The model under review builds one solid part; all positions refer to its coordinate system, in mm. Give positions to 0.01 mm unless a question says otherwise; leave off trailing zeros. Write each loop counter-clockwise with the first axis right and the second up, starting at its lowest first coordinate (ties: lowest second). Pieces come first, ordered by that corner, then holes. Notation, with made-up numbers: (-14, -35) - (-4, -35) arc R14 cw to (-4, -18) - close; hole circle Ø2 at (42, -35). An arc over 180 degrees is marked (long way). Write item = value, one per line.
```python
from build123d import *

# Parameters (mm, degrees)
EXTRUDE_THIN1_DEPTH = 1.2
EXTRUDE_THIN2_DEPTH = 1.2
BOSS_EXTRUDE1_DEPTH = 50.02
EXTRUDE_THIN5_START = -2.6
EXTRUDE_THIN5_DEPTH = 2.6


# Read off the part's stored shape, not the designer's step: Extrude-Thin1
with BuildPart() as part:
    # Extrude-Thin1 outline → Extrude-Thin1 (new body)
    with BuildSketch(Plane(origin=(0, 0, 0), x_dir=(1, 0, 0), z_dir=(0, 1, 0))):
        Polygon((-25.01, 39.998768944), (-15.007807764, -0.01), (15.007807764, -0.01), (25.01, 39.998768944), (25.01, 42.01), (-25.01, 42.01), align=None)
        Polygon((13.594602468, 1.8), (-13.594602468, 1.8), (-23.194602468, 40.2), (23.194602468, 40.2), align=None, mode=Mode.SUBTRACT)
    extrude(amount=EXTRUDE_THIN1_DEPTH)

    # Sketch3 → Extrude-Thin2 (add)
    with BuildSketch(Plane.XZ):
        Polygon((23.844483111, -39.577380413), (-12.944721826, -1.177380413), (-14.244483111, -2.422619587), (22.544721826, -40.822619587), align=None)
        Polygon((-22.544721826, -40.822619587), (14.244483111, -2.422619587), (12.944721826, -1.177380413), (-23.844483111, -39.577380413), align=None)
    extrude(amount=-EXTRUDE_THIN2_DEPTH)

    # Sketch4 → Boss-Extrude1 (add)
    with BuildSketch(Plane.ZY.offset(25.01)):
        with BuildLine():
            Line((-42.326963696, 2.62973084), (-42.83410561, 3.717300185))
            ThreePointArc((-42.83410561, 3.717300185), (-43.913777214, 1.527942753), (-42.01, 0))
            Line((-42.01, 0), (-42.01, 1.2))
            ThreePointArc((-42.01, 1.2), (-42.742222005, 1.78767029), (-42.326963696, 2.62973084))
        make_face()
    extrude(amount=-BOSS_EXTRUDE1_DEPTH)

    # Sketch5 → Extrude-Thin5 (add)
    with BuildSketch(Plane.XZ.offset(EXTRUDE_THIN5_START)):
        Polygon((25.01, -42.01), (25.01, -39.998768944), (15.007807764, 0.01), (-15.007807764, 0.01), (-25.01, -39.998768944), (-25.01, -42.01), (-25.81, -42.01), (-25.81, -39.900284443), (-15.632428889, 0.81), (15.632428889, 0.81), (25.81, -39.900284443), (25.81, -42.01), align=None)
    extrude(amount=EXTRUDE_THIN5_DEPTH)


solid = part.part
```
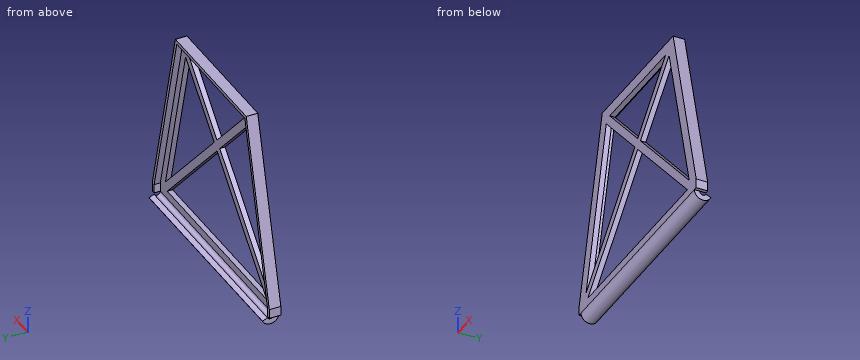
1. For line 1 (X direction, y = 1, z = -36); line 2 (X direction, y = 0.7, z = -22.5); line 3 (Z direction, x = -3, y = 0.3), list the stretches that pass through material, from the lowest coordinate up. Write a range as from..to.
Findings below:
line_1 = -24.83..-22.14, -20.42..-17.92, 17.92..20.42, 22.14..24.83
line_2 = -21.46..-18.77, -7.48..-4.99, 4.99..7.48, 18.77..21.46
line_3 = -43.05..-40.2, -20.42..-17.82, -14.16..-11.56, -1.8..0.81
2. Insertion check: P1, Ø5, axis at x = -9, z = -36.5, coming from the +Y side; P2, Ø0.9, axis at x = -25.5, y = 1.5, coming from the -Z side; P3, Ø2, axis at y = 1, z = -33.5, coming from the -X side; P4, Ø1.5, axis at y = 2.5, z = -28.5, coming from the +X side. Each pin has a flat end and moves straight along its axis. Give the tip position at first contact, or say it passes through.
Findings below:
P1 = through
P2 = -42.01
P3 = -24.46
P4 = 23.15
3. Take a section at A-A on x = 21. Give the boundary of the cut face in (y, z), and give its area (3 significant figures).
Findings below:
outline = (0, -42.01) arc R1.95 ccw to (3.72, -42.83) - (2.63, -42.33) arc R0.75 cw to (1.2, -42.01) - (1.2, -40.2) - (0, -40.2) - close; (0, -39.21) - (1.2, -39.21) - (1.2, -36.61) - (0, -36.61) - close; (0, -31.42) - (1.2, -31.42) - (1.2, -23.96) - (2.6, -23.96) - (2.6, -20.66) - (0, -20.66) - close
area = 27.2 mm²
4. Take a section at D-D on x = 7.5. Give the boundary of the cut face in (y, z).
Findings below:
outline = (0, -42.01) arc R1.95 ccw to (3.72, -42.83) - (2.63, -42.33) arc R0.75 cw to (1.2, -42.01) - (1.2, -40.2) - (0, -40.2) - close; (0, -25.12) - (1.2, -25.12) - (1.2, -22.52) - (0, -22.52) - close; (0, -9.46) - (1.2, -9.46) - (1.2, -6.86) - (0, -6.86) - close; (0, -1.8) - (1.2, -1.8) - (1.2, 0.01) - (2.6, 0.01) - (2.6, 0.81) - (0, 0.81) - close
5. Take a section at C-C on z = -6.5. Give the boundary of the cut face in (x, y), and give its area (3 significant figures).
Findings below:
outline = (-17.46, 0) - (-14.77, 0) - (-14.77, 1.2) - (-16.64, 1.2) - (-16.64, 2.6) - (-17.46, 2.6) - close; (-10.34, 0) - (-7.85, 0) - (-7.85, 1.2) - (-10.34, 1.2) - close; (7.85, 0) - (10.34, 0) - (10.34, 1.2) - (7.85, 1.2) - close; (14.77, 0) - (17.46, 0) - (17.46, 2.6) - (16.64, 2.6) - (16.64, 1.2) - (14.77, 1.2) - close
area = 14.7 mm²
6. Take a section at B-B on y = 1.9. Give the boundary of the cut face in (x, z).
Findings below:
outline = (-25.81, -42.01) - (-25.01, -42.01) - (-25.01, -40) - (-15.01, 0.01) - (15.01, 0.01) - (25.01, -40) - (25.01, -42.01) - (25.81, -42.01) - (25.81, -39.9) - (15.63, 0.81) - (-15.63, 0.81) - (-25.81, -39.9) - close; (-25.01, -43.96) - (25.01, -43.96) - (25.01, -42.76) - (-25.01, -42.76) - close
